Source: CAD feature listing. Evaluate the final solid. Frame: model axes, mm. Face numbers are marked on the shaded views. A direction names the side the tool comes from. Give positions to 0.01 mm unless a question says otherwise; leave off trailing zeros. Loops run counter-clockwise (first coordinate to the right, second up) from the corner with the lowest first, then second, coordinate; pieces in that order, holes last. Notation, with made-up numbers: (7.5, -16.75) - (61.5, -16.75) arc R28 cw to (61.5, 1.25) - close; hole circle Ø1 at (-26.5, 35). An arc over 180 degrees is marked (long way). Put each result on its own line as item: value.
```python
from build123d import *

# Parameters (mm, degrees)
SKETCH_1_W          = 15
SKETCH_1_H          = 15
SKETCH_1_W_2        = 13
SKETCH_1_H_2        = 13
EXTRUDE_1_DEPTH     = 40
SKETCH_2_R          = 1.45
CUT_EXTRUDE_1_DEPTH = 44.373378932


with BuildPart() as part:
    # 草图1 → 凸台-拉伸1 (new body)
    with BuildSketch(Plane(origin=(0, 0, 0), x_dir=(0, 0, -1), z_dir=(1, 0, 0))):
        Rectangle(SKETCH_1_W, SKETCH_1_H)
        Rectangle(SKETCH_1_W_2, SKETCH_1_H_2, mode=Mode.SUBTRACT)
    extrude(amount=EXTRUDE_1_DEPTH)

    # 草图2 → 切除-拉伸1 (cut, through all)
    with BuildSketch(Plane(origin=(0, 7.5, 0), x_dir=(1, 0, 0), z_dir=(0, 1, 0))):
        with Locations(Location((5, 0, 0), (0, 0, 270))):
            Circle(SKETCH_2_R)
        with Locations(Location((25, 0, 0), (0, 0, 270))):
            Circle(SKETCH_2_R)
        with Locations(Location((35, 0, 0), (0, 0, 270))):
            Circle(SKETCH_2_R)
    extrude(amount=-CUT_EXTRUDE_1_DEPTH, mode=Mode.SUBTRACT)


solid = part.part
```
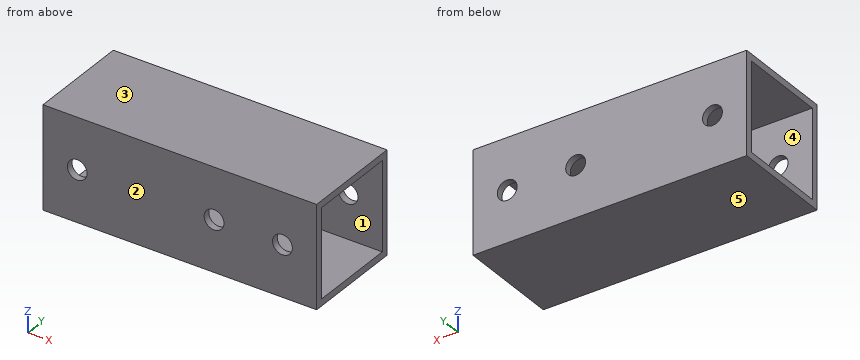
1) Mould query, pull axis Z, two halves, no side actions, for the marked faces 1, 2 and 3. Classes: pulls with the +Z half, pulls with the -Z half, needs draft (parallel to the pull), parting line crosses it, or undercut.
Check result:
face 1: undercut
face 2: needs draft
face 3: pulls with the +Z half
2) Access query for the marked faces 4 and 5. Directions: +Z, -Z, +X, -X, +Y, -Y. A direction counts if a zero-diameter tool reaches every point of the face in a straight line with its end or side. Return the directions, or none.
Check result:
face 4: +X, -X
face 5: -Z, +X, -X, +Y, -Y
3) Section query A-A, the plane y = -5. Output: boundary loops of the cut face in (x, z).
Check result:
outline: (0, -7.5) - (40, -7.5) - (40, -6.5) - (0, -6.5) - close; (0, 6.5) - (40, 6.5) - (40, 7.5) - (0, 7.5) - close
4) Section query D-D, the plane z = 0. State how many separate pieces and enclosed holes the cut face has, plus the area to 3 significant figures.
Check result:
separate pieces: 8
enclosed holes: 0
area: 62.6 mm²
5) Material intervals for line 1 along X through (y, z) = (7, 0); line 2 along Y through (x, z) = (25.5, -3.5), sorted ascending. Write a range as [from, to].
Check result:
line 1: [0, 3.55], [6.45, 23.55], [26.45, 33.55], [36.45, 40]
line 2: [-7.5, -6.5], [6.5, 7.5]
6) Pin query (flat end, axial travel): P1, Ø2.5, axis at x = 5, z = 0, coming from the +Y side. Return the tip coordinate at first contact, or that it passes through.
Check result:
P1: through
7) Section query C-C, the plane x = 5. Output: boundary loops of the cut face in (y, z).
Check result:
outline: (-7.5, -7.5) - (7.5, -7.5) - (7.5, -1.45) - (6.5, -1.45) - (6.5, -6.5) - (-6.5, -6.5) - (-6.5, -1.45) - (-7.5, -1.45) - close; (-7.5, 1.45) - (-6.5, 1.45) - (-6.5, 6.5) - (6.5, 6.5) - (6.5, 1.45) - (7.5, 1.45) - (7.5, 7.5) - (-7.5, 7.5) - close
